Autodesk Inventor part; units mm, degrees
ref_plane "Work Plane1" through (7.5, 0, 0) normal (1, 0, 0) x (0, 1, 0)
ref_plane "XZ Plane" through (0, 0, 0) normal (0, 1, 0) x (-1, 0, 0)
ref_plane "XY Plane" through (0, 0, 0) normal (0, 0, 1) x (1, 0, 0)
sketch "Sketch1" plane through (0, 0, 0) normal (0, 0, 1) x (1, 0, 0)
  circle A0 centre (0, 0) radius 7.5
  dimension "d0" = 15
extrude "Extrusion1" add sketch "Sketch1" along normal blind 205.029
sketch "Sketch2" plane through (0, 0, 205.029) normal (0, 0, 1) x (1, 0, 0)
  point P0 (0, 0)
  point P1 (-0.1268, -0.0213)
hole "Hole1" at (-0.1268, -0.0213, 205.029) direction (0, 0, -1) diameter 7 end through all
ref_plane "Work Plane1" through (7.5, 0, 0) normal (1, 0, 0) x (0, 1, 0)
sketch "Sketch3" plane through (7.5, 0, 0) normal (1, 0, 0) x (0, 1, 0)
  circle A0 centre (0, 198.029) radius 1
  line L0 (7.5, 205.029) -> (-7.5, 205.029)
  point P0 (0, 0)
  dimension "d10" = 2
  dimension "d11" = 7
extrude "Extrusion2" cut sketch "Sketch3" against normal through all
properties part number "shaft" material "Nylon 6/6"
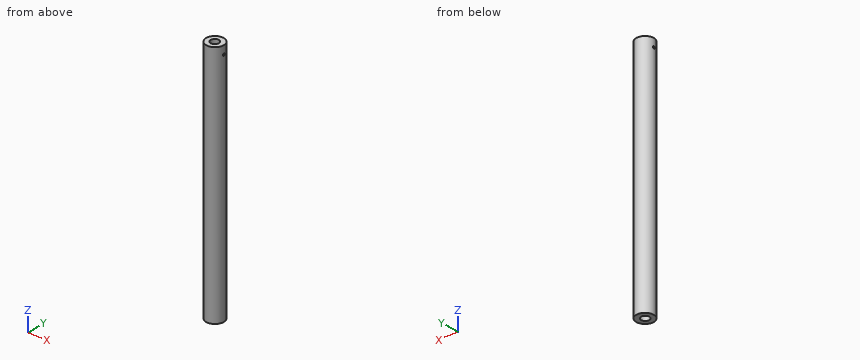
Input: part model. Units: mm. Frame: model coordinates. Coordinates: 2 decimals unless noted, no trailing zeros. Loops run counter-clockwise (first coordinate to the right, second up) from the corner with the lowest first, then second, coordinate; pieces in that order, holes last.
(1) Section A-A on z = 93. Return the cut outline in (x, y).
(2) Material intervals for probe 1 along Z at (x, y) = (3.75, 0); probe 2 along Y at (x, z) = (1.25, 175); probe 3 along X at (y, z) = (1.5, 115.5), sorted ascending.
(3) First-contact query: pin 1 Ø4 at (x, z) = (3, 130.5) entering from +Y; pin 2 Ø3 at (y, z) = (-1, 170.5) entering from +X; pin 3 Ø3 at (y, z) = (5.5, 87) entering from -X; pin 4 Ø3 at (y, z) = (3.5, 175) entering from -X. Flat tips, straight axial feed; report the tip coordinate or a pass-through.
(4) Section B-B on x = 5.25. Return the cut outline in (y, z), then the cut area to 3 significant figures.
(5) Section C-C on y = 5.75. Return the cut outline in (x, z).
Data:
1. outline: circle Ø15 at (0, 0); hole circle Ø7 at (-0.13, -0.02)
2. probe 1: z = 0 to 197.03, 199.03 to 205.03
2. probe 2: y = -7.4 to -3.24, 3.2 to 7.4
2. probe 3: x = -7.35 to -3.28, 3.03 to 7.35
3. pin 1: stops at y = 7.43
3. pin 2: stops at x = 7.5
3. pin 3: stops at x = -6.34
3. pin 4: stops at x = -7.23
4. outline: (-5.36, 0) - (5.36, 0) - (5.36, 205.03) - (-5.36, 205.03) - close; hole circle Ø2 at (0, 198.03)
4. area: 2,190 mm2
5. outline: (-4.82, 0) - (4.82, 0) - (4.82, 205.03) - (-4.82, 205.03) - close
